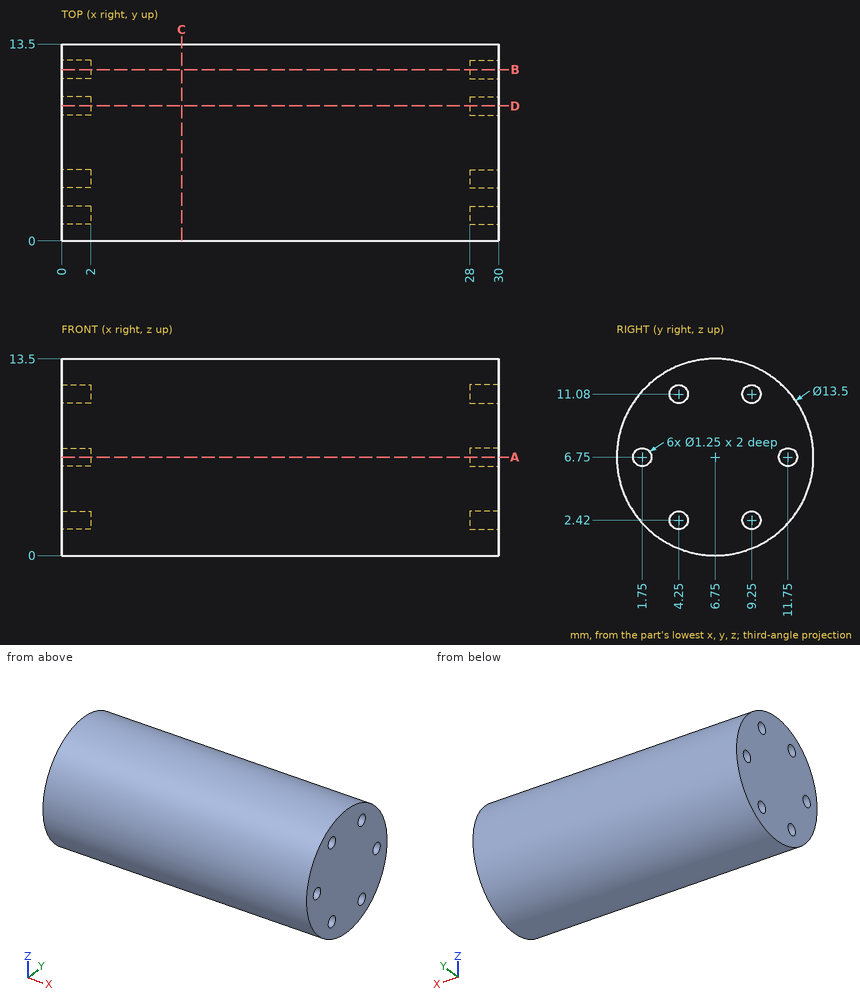
The drawing under review shows one solid part. Ordinate dimensions are in mm from its lowest x, y, z. Coordinates: 2 decimals unless noted, no trailing zeros. Write each loop counter-clockwise with the first axis right and the second up, starting at its lowest first coordinate (ties: lowest second). Pieces come first, ordered by that corner, then holes.
1) Add section B-B (y = 11.75). Write out the cut boundary in (x, z) (1 decimal), plus the area to 3 significant figures.
2) To check wall thickness, follow L1, parallel to Y at x = 29.3, z = 6.75 (3 decimals); L2, parallel to Y at x = 6, z = 3; L3, parallel to Y at x = 24.25, z = 5.5. State the ranges of each line that lie inside material, in increasing order.
3) Add section A-A (z = 6.75). Write out the cut boundary in (x, y) (3 decimals).
4) Add section C-C (x = 8.25). Write out the cut boundary in (y, z), plus the area to 3 significant figures.
5) Insertion check: pin 1 (0.8 mm diameter, centred on y = 4.25, z = 11.08, fed in from -X); pin 2 (2 mm diameter, centred on x = 17, y = 12, fed in from +Z); pin 3 (2 mm diameter, centred on x = 16, y = 8.5, fed in from -Z). Each pin has a flat end and moves straight along its axis. Give the tip position at first contact, or say it passes through.
6) Add section D-D (y = 9.25). Write out the cut boundary in (x, z) (3 decimals).
Check result:
1. outline: (0, 2.2) - (30, 2.2) - (30, 6.1) - (28, 6.1) - (28, 7.4) - (30, 7.4) - (30, 11.3) - (0, 11.3) - (0, 7.4) - (2, 7.4) - (2, 6.1) - (0, 6.1) - close
1. area: 267 mm2
2. L1: y = 0 to 1.125, 2.375 to 11.125, 12.375 to 13.5
2. L2: y = 1.14 to 12.36
2. L3: y = 0.12 to 13.38
3. outline: (0, 0) - (30, 0) - (30, 1.125) - (28, 1.125) - (28, 2.375) - (30, 2.375) - (30, 11.125) - (28, 11.125) - (28, 12.375) - (30, 12.375) - (30, 13.5) - (0, 13.5) - (0, 12.375) - (2, 12.375) - (2, 11.125) - (0, 11.125) - (0, 2.375) - (2, 2.375) - (2, 1.125) - (0, 1.125) - close
4. outline: circle Ø13.5 at (6.75, 6.75)
4. area: 143 mm2
5. pin 1: stops at x = 2
5. pin 2: stops at z = 11.99
5. pin 3: stops at z = 0.04
6. outline: (0, 0.48) - (30, 0.48) - (30, 1.795) - (28, 1.795) - (28, 3.045) - (30, 3.045) - (30, 10.455) - (28, 10.455) - (28, 11.705) - (30, 11.705) - (30, 13.02) - (0, 13.02) - (0, 11.705) - (2, 11.705) - (2, 10.455) - (0, 10.455) - (0, 3.045) - (2, 3.045) - (2, 1.795) - (0, 1.795) - close
